The drawing under review shows one solid part. Ordinate dimensions are in mm from its lowest x, y, z. Give positions to 0.01 mm unless a question says otherwise; leave off trailing zeros. Loops run counter-clockwise (first coordinate to the right, second up) from the corner with the lowest first, then second, coordinate; pieces in that order, holes last. Notation, with made-up numbers: M 17,62 L 40,62 A17 ccw 40,92 Z; hole C 15.25,-32.5 d9. An arc over 180 degrees is marked long. One line per item, written item: value. Start each with the question number.
Q1. We need section C-C on z = 74. Write out the cut boundary in (x, y).
Q2. For pin 1 (12 mm diameter, centred on x = 27, z = 84.5, fed in from -Y); pin 2 (3 mm diameter, centred on x = 24, y = 22, fed in from +Z), all flat-tipped, find the tip position at first contact; note any pin that passes through.
Q3. To check wall thickness, follow line 1 along Z through (x, y) = (10.5, 8) (1 decimal); line 2 along Z through (x, y) = (34, 7); line 3 along X through (y, z) = (15, 69). State the ranges of each line that lie inside material, in increasing order. Write a range as from..to.
Q4. We need section B-B on x = 3.5. Write out the cut boundary in (y, z), plus the area to 3 significant figures.
Q5. We need section A-A on y = 30.5. Write out the cut boundary in (x, z), plus the area to 3 significant figures.
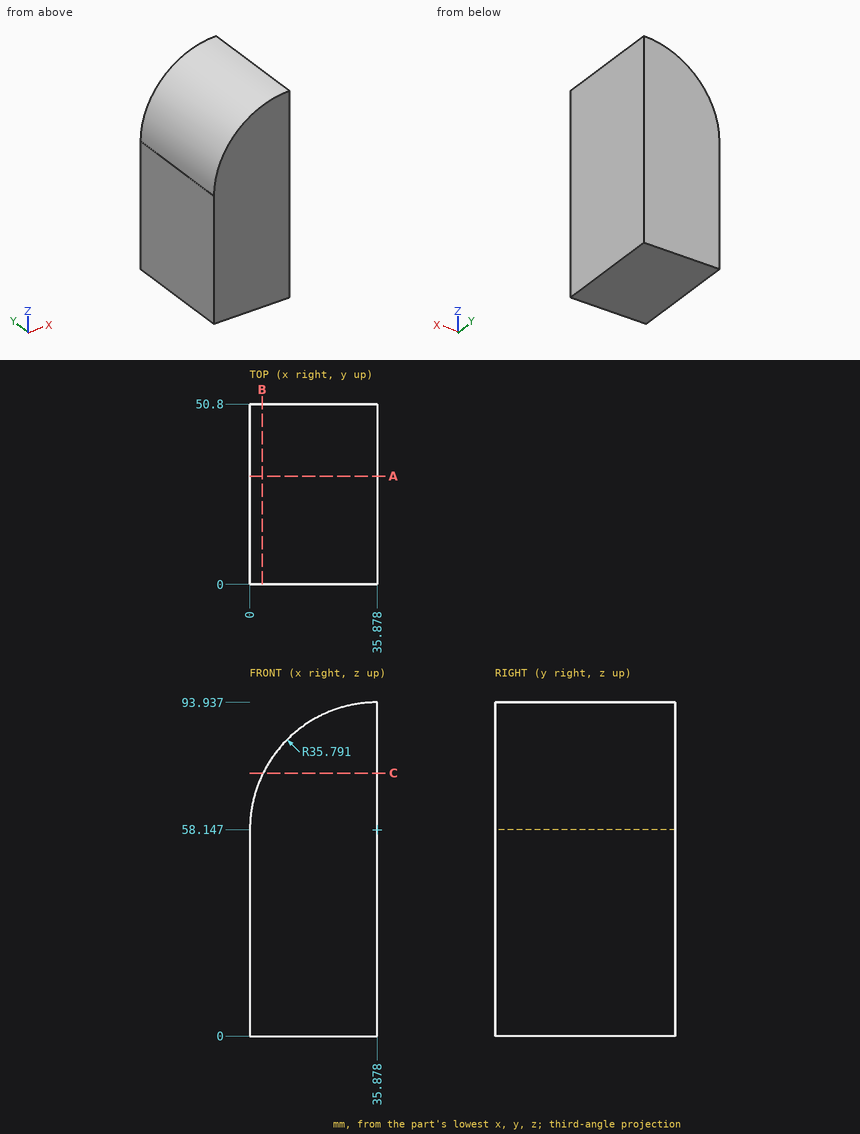
Solved:
1. outline: M 3.79,0 L 35.88,0 L 35.88,50.8 L 3.79,50.8 Z
2. pin 1: y = 0
2. pin 2: z = 92.4
3. line 1: 0..83.4
3. line 2: 0..93.89
3. line 3: 1.77..35.88
4. outline: M 0,0 L 50.8,0 L 50.8,73.4 L 0,73.4 Z
4. area: 3,730 mm2
5. outline: M 0,0 L 35.88,0 L 35.88,93.94 A35.79 ccw 0.09,58.15 L 0,58.15 Z
5. area: 3,090 mm2
